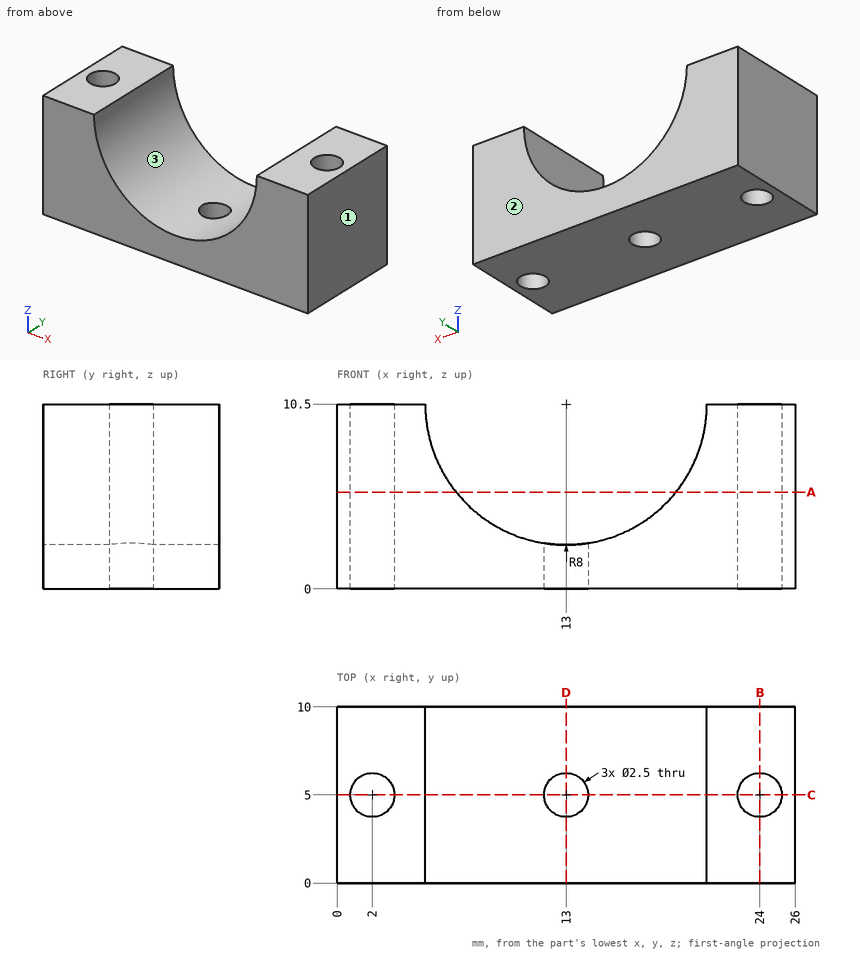
Here's the drawing with two shaded views (mm, measured from the low corner). I have some questions. Give positions to 0.01 mm unless a question says otherwise; leave off trailing zeros. Loops run counter-clockwise (first coordinate to the right, second up) from the corner with the lowest first, then second, coordinate; pieces in that order, holes last. Notation, with made-up numbers: M 75,0 L 134,0 A35 ccw 134,38 Z; hole C 31.5,5 d2. An arc over 180 degrees is marked long. Use one line per item in the form item = value. Start each with the question number.
Q1. If we section it at B-B (x = 24): Write out the boundary of the cut face in (y, z).
Q2. Will this pin go through, and if not, where does the flat tip stop? pin 1 Ø5 at (y, z) = (3, 4.5) entering from -X.
Q3. If we section it at D-D (x = 13): Write out the boundary of the cut face in (y, z).
Q4. Thinking about a two-plate mould opening in X: for the marked faces 1, 2 and 3, which applies, +X half, -X half, draft (parallel to the pull), parting line (faces both ways), or undercut?
Q5. If we section it at C-C (y = 5): Write out the boundary of the cut face in (x, z), then the cut area to 3 significant figures.
Q6. I need wall thicknesses on line 1 along Y through (x, z) = (24, 8.25); line 2 along X through (y, z) = (5.5, 0.5); line 3 along X through (y, z) = (5.75, 6.25). Which ranges of each line are inside material? Lowest first, please.
Q7. If we section it at A-A (z = 5.5): Write out the boundary of the cut face in (x, y) (3 decimals).
Taken from the geometry:
q1.outline = M 0,0 L 3.75,0 L 3.75,10.5 L 0,10.5 Z; M 6.25,0 L 10,0 L 10,10.5 L 6.25,10.5 Z
q2.pin_1 = 0
q3.outline = M 0,0 L 3.75,0 L 3.75,2.5 L 0,2.5 Z; M 6.25,0 L 10,0 L 10,2.5 L 6.25,2.5 Z
q4.face_1 = +X half
q4.face_2 = draft
q4.face_3 = undercut
q5.outline = M 0,0 L 0.75,0 L 0.75,10.5 L 0,10.5 Z; M 3.25,0 L 11.75,0 L 11.75,2.6 A8 cw 5,10.5 L 3.25,10.5 Z; M 14.25,0 L 22.75,0 L 22.75,10.5 L 21,10.5 A8 cw 14.25,2.6 Z; M 25.25,0 L 26,0 L 26,10.5 L 25.25,10.5 Z
q5.area = 114 mm^2
q6.line_1 = 0 to 3.75, 6.25 to 10
q6.line_2 = 0 to 0.85, 3.15 to 11.85, 14.15 to 22.85, 25.15 to 26
q6.line_3 = 0 to 1, 3 to 6.22, 19.78 to 23, 25 to 26
q7.outline = M 0,0 L 6.755,0 L 6.755,10 L 0,10 Z; M 19.245,0 L 26,0 L 26,10 L 19.245,10 Z; hole C 2,5 d2.5; hole C 24,5 d2.5
